Part model, mm, in its own coordinate system. Coordinates: 2 decimals unless noted, no trailing zeros. Order: outer loops, then holes, each group sorted by start corner. A loop starts at its lowest first (then second) coordinate and runs counter-clockwise, first axis right, second up. Notation, with made-up numbers: (4, 55) - (38, 55) arc R18 ccw to (38, 69) - close; hole circle Ø8 at (-14.75, 56.5). An arc over 180 degrees is marked (long way). Use a Markdown table: item, result. Add a question column.
1) Saw through at C-C on z = 30. List the corners of the cut face in (x, y).
2) Saw through at B-B on x = -55. List the corners of the cut face in (y, z), then the cut area to 3 significant figures.
3) Drop a flat-ended pin along its axis: P1, Ø6, axis at x = -58.5, z = 30, coming from the -Y side. Give the stop position or say it passes through.
4) Wall check: L1, parallel to Y at x = -52.5, z = 33; L2, parallel to Y at x = -51, z = 36.75. Give the ranges that are in metal, low to high. Write a range as [from, to].
5) Saw through at D-D on x = -60.5. List the corners of the cut face in (y, z), then the cut area to 3 significant figures.
6) Two-plate mould, pull along X, no slides. Class faces 1 (the face through (-53, -108.804, 28)), 2 (the face through (-42.976, -44, 28)), 3 (the face through (-49.07, -101.48, 28.44)): +X half, -X half, draft (parallel to the pull), parting line (faces both ways), or undercut.
7) Saw through at A-A on y = -101.5. List the corners of the cut face in (x, z), then the cut area to 3 significant figures.
Solid Edge part; units mm, degrees
sketch "Sketch1" plane through (0, 0, 0) normal (0, -1, 0) x (1, 0, 0)
  line L0 (-62.9763, 18.5767) -> (-42.9763, 18.5767)
  line L1 (-42.9763, 18.5767) -> (-42.9763, 38.5767)
  line L2 (-42.9763, 38.5767) -> (-62.9763, 38.5767)
  line L3 (-62.9763, 38.5767) -> (-62.9763, 18.5767)
extrude "Protrusion1" add sketch "Sketch1" along normal blind 90
sketch "Sketch2" plane through (-52.9763, -30, 18.5767) normal (0, 0, -1) x (0, -1, 0)
  circle A0 centre (72.3427, 0) radius 4
  line L0 (60, 10) -> (78.8043, 3.7638)
  line L1 (78.8043, 3.7638) -> (78.8043, -3.7638)
  line L2 (78.8043, -3.7638) -> (60, -10)
  line L3 (60, -10) -> (60, 10)
extrude "Protrusion2" add sketch "Sketch2" against normal up to vertex (20 mm away)
Results are:
| question | item | result |
|---|---|---|
| 1 | outline | (-62.98, -90) - (-56.74, -108.8) - (-49.21, -108.8) - (-42.98, -90) - (-42.98, 0) - (-62.98, 0) - close; hole circle Ø8 at (-52.98, -102.34) |
| 2 | outline | (-108.8, 18.58) - (-105.79, 18.58) - (-105.79, 38.58) - (-108.8, 38.58) - close; (-98.89, 18.58) - (0, 18.58) - (0, 38.58) - (-98.89, 38.58) - close |
| 2 | area | 2,040 mm2 |
| 3 | P1 | y = -108.8 |
| 4 | L1 | [-108.8, -106.31], [-98.37, 0] |
| 4 | L2 | [-108.8, -105.82], [-98.87, 0] |
| 5 | outline | (-97.47, 18.58) - (0, 18.58) - (0, 38.58) - (-97.47, 38.58) - close |
| 5 | area | 1,950 mm2 |
| 6 | face 1 | draft |
| 6 | face 2 | +X half |
| 6 | face 3 | undercut |
| 7 | outline | (-59.16, 18.58) - (-56.89, 18.58) - (-56.89, 38.58) - (-59.16, 38.58) - close; (-49.07, 18.58) - (-46.79, 18.58) - (-46.79, 38.58) - (-49.07, 38.58) - close |
| 7 | area | 91.0 mm2 |
